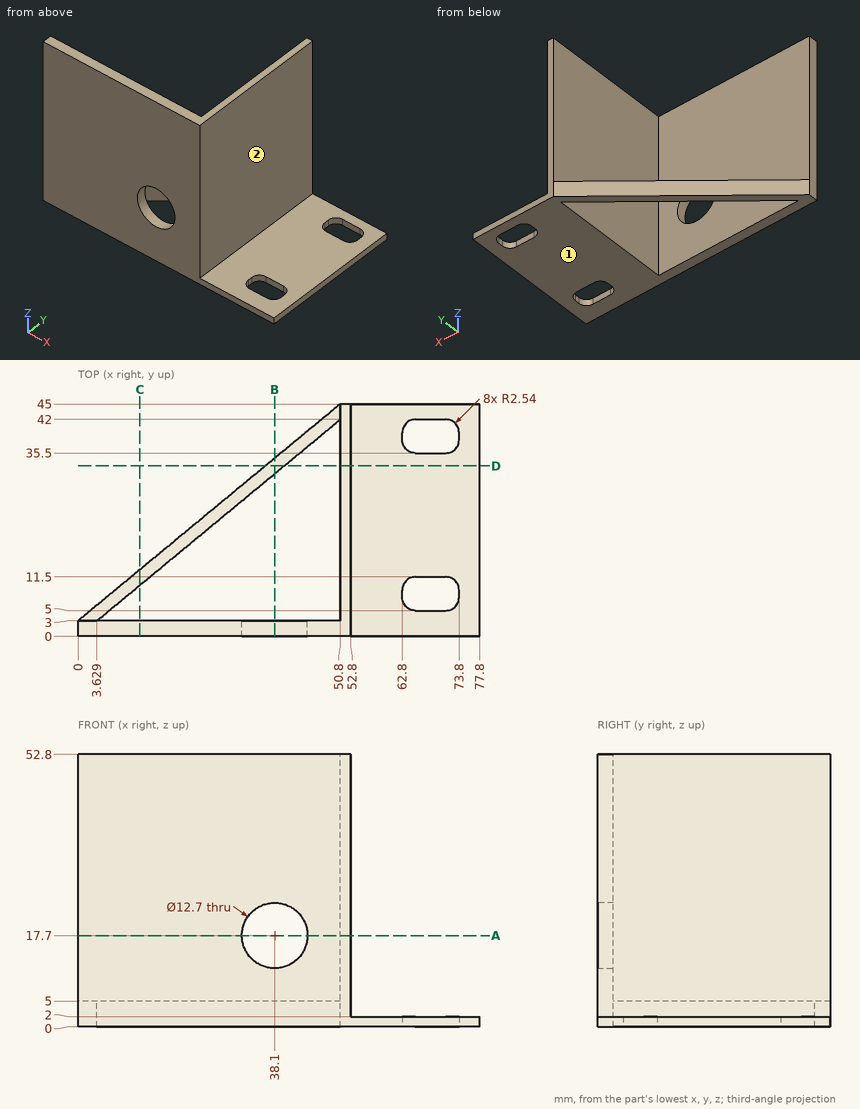
Study the drawing (mm; zero at the part's minimum x, y, z) and answer. A direction names the side the tool comes from. Coordinates: 2 decimals unless noted, no trailing zeros. Loops run counter-clockwise (first coordinate to the right, second up) from the corner with the lowest first, then second, coordinate; pieces in that order, holes last. Notation, with made-up numbers: M 39.25,-14 L 81.25,-14 A13 ccw 81.25,8 Z; hole C 23.5,58 d3. An arc over 180 degrees is marked long. Answer in a Markdown table with one row per item. Add a question column.
1. Find section A-A, the plane z = 17.7. Write down the section's boundary in (x, y).
2. A tool of negligible diameter and unlimited length cuts with its end or side. For the marked faces 1 and 2, from which of +Z, -Z, +X, -X, +Y, -Y can it reach the whole face along a straight path? Write none if from no direction.
3. Find section C-C, the plane x = 12. Write down the section's boundary in (y, z).
4. Flat-ended cylindrical pins translate along their axes: P1, Ø4, axis at x = 55.5, z = 30, coming from the -Y side; P2, Ø1.6, axis at y = 8, z = 1.5, coming from the -X side; P3, Ø7.5, axis at x = 69, y = 19, coming from the +Z side; P4, Ø1.6, axis at y = 39, z = 1, coming from the -X side (1 decimal). Find the tip coordinate at first contact, or state that the pin passes through.
5. Consider L1, parallel to X at y = 1.6, z = 17.7; L2, parallel to Y at x = 26.5, z = 44.5; L3, parallel to X at y = 30.5, z = 20. Determine where each line is inside the solid, lowest interval first.
6. Find section D-D, the plane y = 33. Write down the section's boundary in (x, z) (1 decimal).
7. Find section B-B, the plane x = 38.1. Write down the section's boundary in (y, z), then the cut area to 3 significant figures.
Reported:
| question | item | result |
|---|---|---|
| 1 | outline | M 0,0 L 31.75,0 L 31.75,3 L 0,3 Z; M 44.45,0 L 52.8,0 L 52.8,45 L 50.8,45 L 50.8,3 L 44.45,3 Z |
| 2 | face 1 | -Z, +X, -X, +Y, -Y |
| 2 | face 2 | +Z, +X, +Y, -Y |
| 3 | outline | M 0,0 L 3,0 L 3,52.8 L 0,52.8 Z; M 9.92,0 L 12.92,0 L 12.92,5 L 9.92,5 Z |
| 4 | P1 | passes through |
| 4 | P2 | stops at x = 5.08 |
| 4 | P3 | stops at z = 2 |
| 4 | P4 | stops at x = 42.6 |
| 5 | L1 | x = 0 to 31.75, 44.45 to 52.8 |
| 5 | L2 | y = 0 to 3 |
| 5 | L3 | x = 50.8 to 52.8 |
| 6 | outline | M 36.3,0 L 39.9,0 L 39.9,5 L 36.3,5 Z; M 50.8,0 L 77.8,0 L 77.8,2 L 52.8,2 L 52.8,52.8 L 50.8,52.8 Z |
| 7 | outline | M 0,0 L 3,0 L 3,11.35 L 0,11.35 Z; M 0,24.05 L 3,24.05 L 3,52.8 L 0,52.8 Z; M 31.5,0 L 34.5,0 L 34.5,5 L 31.5,5 Z |
| 7 | area | 135 mm^2 |
